from build123d import *

# Parameters (mm, degrees)
SKETCH1_R           = 1.75
BOSS_EXTRUDE1_DEPTH = 13
BOSS_EXTRUDE2_START = -2.8
BOSS_EXTRUDE2_DEPTH = 2.8
CIRPATTERN1_START   = 10.2
CIRPATTERN1_DEPTH   = 2.8


# Read off the part's stored shape, not the designer's step: CirPattern1
with BuildPart() as part:
    # Sketch1 → Boss-Extrude1 (new body)
    with BuildSketch(Plane.XY):
        with Locations(Location((0, 0, 0), (0, 0, 180))):
            Circle(SKETCH1_R)
    extrude(amount=BOSS_EXTRUDE1_DEPTH)

    # Sketch2 → Boss-Extrude2 (add)
    with BuildSketch(Plane.XY.offset(13).offset(BOSS_EXTRUDE2_START)):
        with BuildLine():
            Line((0.095027487, 1.747418031), (0, 1.941449497))
            Line((0, 1.941449497), (-0.099072162, 1.74719338))
            ThreePointArc((-0.099072162, 1.74719338), (-0.002025455, 1.749998828), (0.095027487, 1.747418031))
        make_face()
    extrude(amount=BOSS_EXTRUDE2_DEPTH)

    # CirPattern1 outline → CirPattern1 (add)
    with BuildSketch(Plane.XY.offset(CIRPATTERN1_START)):
        with BuildLine():
            Line((-0.360475563, 1.712471129), (-0.502484105, 1.87529621))
            Line((-0.502484105, 1.87529621), (-0.547903282, 1.662017447))
            ThreePointArc((-0.547903282, 1.662017447), (-0.454889465, 1.689844838), (-0.360475563, 1.712471129))
        make_face()
        with BuildLine():
            Line((0.502484105, 1.87529621), (0.356510562, 1.713300972))
            ThreePointArc((0.356510562, 1.713300972), (0.450976586, 1.69089329), (0.54405457, 1.663281283))
            Line((0.54405457, 1.663281283), (0.502484105, 1.87529621))
        make_face()
        with BuildLine():
            ThreePointArc((-0.959395699, 1.463577771), (-0.876753509, 1.514530714), (-0.791412798, 1.56082215))
            Line((-0.791412798, 1.56082215), (-0.970724749, 1.681344585))
            Line((-0.970724749, 1.681344585), (-0.959395699, 1.463577771))
        make_face()
        with BuildLine():
            Line((0.970724749, 1.681344585), (0.787797681, 1.562649933))
            ThreePointArc((0.787797681, 1.562649933), (0.873245319, 1.516556169), (0.956005233, 1.465794663))
            Line((0.956005233, 1.465794663), (0.970724749, 1.681344585))
        make_face()
        with BuildLine():
            ThreePointArc((-1.305506884, 1.165397689), (-1.238868251, 1.236003826), (-1.168416559, 1.30280572))
            Line((-1.168416559, 1.30280572), (-1.372812105, 1.372812105))
            Line((-1.372812105, 1.372812105), (-1.305506884, 1.165397689))
        make_face()
        with BuildLine():
            Line((1.372812105, 1.372812105), (1.165397689, 1.305506884))
            ThreePointArc((1.165397689, 1.305506884), (1.236003826, 1.238868251), (1.30280572, 1.168416559))
            Line((1.30280572, 1.168416559), (1.372812105, 1.372812105))
        make_face()
        with BuildLine():
            ThreePointArc((-1.562649933, 0.787797681), (-1.516556169, 0.873245319), (-1.465794663, 0.956005233))
            Line((-1.465794663, 0.956005233), (-1.681344585, 0.970724749))
            Line((-1.681344585, 0.970724749), (-1.562649933, 0.787797681))
        make_face()
        with BuildLine():
            Line((1.681344585, 0.970724749), (1.463577771, 0.959395699))
            ThreePointArc((1.463577771, 0.959395699), (1.514530714, 0.876753509), (1.56082215, 0.791412798))
            Line((1.56082215, 0.791412798), (1.681344585, 0.970724749))
        make_face()
        with BuildLine():
            ThreePointArc((-1.713300972, 0.356510562), (-1.69089329, 0.450976586), (-1.663281283, 0.54405457))
            Line((-1.663281283, 0.54405457), (-1.87529621, 0.502484105))
            Line((-1.87529621, 0.502484105), (-1.713300972, 0.356510562))
        make_face()
        with BuildLine():
            Line((1.87529621, 0.502484105), (1.662017447, 0.547903282))
            ThreePointArc((1.662017447, 0.547903282), (1.689844838, 0.454889465), (1.712471129, 0.360475563))
            Line((1.712471129, 0.360475563), (1.87529621, 0.502484105))
        make_face()
        with BuildLine():
            ThreePointArc((-1.74719338, -0.099072162), (-1.749998828, -0.002025455), (-1.747418031, 0.095027487))
            Line((-1.747418031, 0.095027487), (-1.941449497, 0))
            Line((-1.941449497, 0), (-1.74719338, -0.099072162))
        make_face()
        with BuildLine():
            Line((1.941449497, 0), (1.74719338, 0.099072162))
            ThreePointArc((1.74719338, 0.099072162), (1.749998828, 0.002025455), (1.747418031, -0.095027487))
            Line((1.747418031, -0.095027487), (1.941449497, 0))
        make_face()
        with BuildLine():
            ThreePointArc((-1.662017447, -0.547903282), (-1.689844838, -0.454889465), (-1.712471129, -0.360475563))
            Line((-1.712471129, -0.360475563), (-1.87529621, -0.502484105))
            Line((-1.87529621, -0.502484105), (-1.662017447, -0.547903282))
        make_face()
        with BuildLine():
            ThreePointArc((-1.463577771, -0.959395699), (-1.514530714, -0.876753509), (-1.56082215, -0.791412798))
            Line((-1.56082215, -0.791412798), (-1.681344585, -0.970724749))
            Line((-1.681344585, -0.970724749), (-1.463577771, -0.959395699))
        make_face()
        with BuildLine():
            Line((1.87529621, -0.502484105), (1.713300972, -0.356510562))
            ThreePointArc((1.713300972, -0.356510562), (1.69089329, -0.450976586), (1.663281283, -0.54405457))
            Line((1.663281283, -0.54405457), (1.87529621, -0.502484105))
        make_face()
        with BuildLine():
            ThreePointArc((-1.165397689, -1.305506884), (-1.236003826, -1.238868251), (-1.30280572, -1.168416559))
            Line((-1.30280572, -1.168416559), (-1.372812105, -1.372812105))
            Line((-1.372812105, -1.372812105), (-1.165397689, -1.305506884))
        make_face()
        with BuildLine():
            Line((1.681344585, -0.970724749), (1.562649933, -0.787797681))
            ThreePointArc((1.562649933, -0.787797681), (1.516556169, -0.873245319), (1.465794663, -0.956005233))
            Line((1.465794663, -0.956005233), (1.681344585, -0.970724749))
        make_face()
        with BuildLine():
            ThreePointArc((-0.787797681, -1.562649933), (-0.873245319, -1.516556169), (-0.956005233, -1.465794663))
            Line((-0.956005233, -1.465794663), (-0.970724749, -1.681344585))
            Line((-0.970724749, -1.681344585), (-0.787797681, -1.562649933))
        make_face()
        with BuildLine():
            Line((1.372812105, -1.372812105), (1.305506884, -1.165397689))
            ThreePointArc((1.305506884, -1.165397689), (1.238868251, -1.236003826), (1.168416559, -1.30280572))
            Line((1.168416559, -1.30280572), (1.372812105, -1.372812105))
        make_face()
        with BuildLine():
            ThreePointArc((-0.356510562, -1.713300972), (-0.450976586, -1.69089329), (-0.54405457, -1.663281283))
            Line((-0.54405457, -1.663281283), (-0.502484105, -1.87529621))
            Line((-0.502484105, -1.87529621), (-0.356510562, -1.713300972))
        make_face()
        with BuildLine():
            Line((0.970724749, -1.681344585), (0.959395699, -1.463577771))
            ThreePointArc((0.959395699, -1.463577771), (0.876753509, -1.514530714), (0.791412798, -1.56082215))
            Line((0.791412798, -1.56082215), (0.970724749, -1.681344585))
        make_face()
        with BuildLine():
            ThreePointArc((0.099072162, -1.74719338), (0.002025455, -1.749998828), (-0.095027487, -1.747418031))
            Line((-0.095027487, -1.747418031), (0, -1.941449497))
            Line((0, -1.941449497), (0.099072162, -1.74719338))
        make_face()
        with BuildLine():
            Line((0.502484105, -1.87529621), (0.547903282, -1.662017447))
            ThreePointArc((0.547903282, -1.662017447), (0.454889465, -1.689844838), (0.360475563, -1.712471129))
            Line((0.360475563, -1.712471129), (0.502484105, -1.87529621))
        make_face()
    extrude(amount=CIRPATTERN1_DEPTH)


solid = part.part
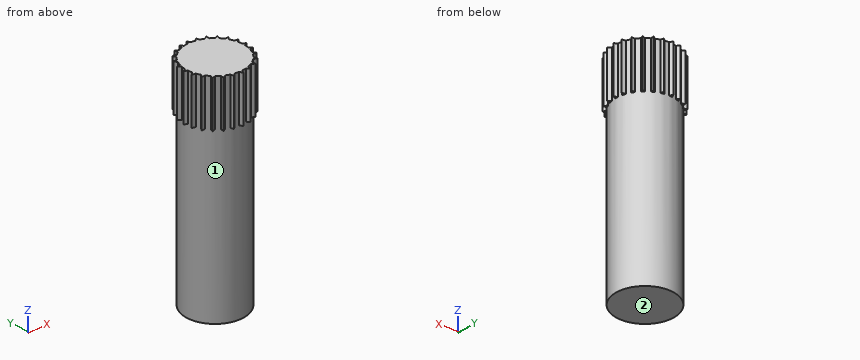
Build history of the part. All positions in model axes, mm. Face numbers are marked on the shaded views. A direction names the side the tool comes from. Coordinates: 2 decimals unless noted, no trailing zeros. Order: outer loops, then holes, each group sorted by start corner. A loop starts at its lowest first (then second) coordinate and runs counter-clockwise, first axis right, second up. Notation, with made-up numbers: M -35,42 L -21,42 A10 ccw -21,51 Z; hole C 3.25,74.5 d7. An arc over 180 degrees is marked long. One line per question, with ' | ' between items. Start each with the question number.
Q1. Flat gauge pins, fed straight in: pin 1 Ø2 at (x, y) = (0.5, -0.5) entering from -Z; pin 2 Ø2 at (y, z) = (1, 5) entering from +X. Where does each tip first touch, or does it go through?
Q2. Saw through at A-A (z = 3.5). List the corners of the cut face in (x, y), then the cut area to 3 significant figures.
Q3. Probe L1, parallel to X at y = -0.55, z = 9.25; L2, parallel to X at y = -1.3, z = 0.5; L3, parallel to Y at x = -0.15, z = 2. List the from-to ranges inside material, lowest first. Write a range as from..to.
Q4. 3-axis set-ups, long thin cutter, end or side, ignore diameter. For the marked faces 1 and 2: which of +Z, -Z, +X, -X, +Y, -Y reach the whole face in a straight line?
Check values:
1) pin 1: stops at z = 0 | pin 2: stops at x = 1.75
2) outline: C 0,0 d3.5 | area: 9.62 mm2
3) L1: x = -1.66..1.66 | L2: x = -1.17..1.17 | L3: y = -1.74..1.74
4) face 1: -Z | face 2: -Z, +X, -X, +Y, -Y
